from build123d import *

# Parameters (mm, degrees)
F0_W     = 1.25
F0_H     = 45
F1_DEPTH = 10
F0_W_2   = 3.75
F2_DEPTH = 2.5
F3_R     = 2.5
F4_R     = 2.5


with BuildPart() as f1:
    # F0 (on Top) → F1 (new body)
    with BuildSketch(Plane.XY):
        with Locations((-0.625, 45)):
            Rectangle(F0_W, F0_H)
        with Locations((0.625, 45)):
            Rectangle(F0_W, F0_H)
        with Locations((-0.625, 0)):
            Rectangle(F0_W, F0_H)
        with Locations((0.625, 0)):
            Rectangle(F0_W, F0_H)
    extrude(amount=F1_DEPTH)

    # F0 (on Top) → F2 (join)
    with BuildSketch(Plane.XY):
        with Locations((3.125, 0)):
            Rectangle(F0_W_2, F0_H)
        with Locations((-3.125, 0)):
            Rectangle(F0_W_2, F0_H)
        with Locations((0.625, 0)):
            Rectangle(F0_W, F0_H)
        with Locations((-0.625, 0)):
            Rectangle(F0_W, F0_H)
    extrude(amount=F2_DEPTH)

    # F3
    f3_edges = [f1.edges().sort_by_distance(p)[0] for p in [
        (5, 22.5, 1.25),
        (-5, 22.5, 1.25),
        (-5, -22.5, 1.25),
        (5, -22.5, 1.25),
    ]]
    fillet(f3_edges, radius=F3_R)

    # F4
    f4_edges = [f1.edges().sort_by_distance(p)[0] for p in [
        (0, -22.5, 10),
        (0, 67.5, 10),
    ]]
    fillet(f4_edges, radius=F4_R)


solid = f1.part
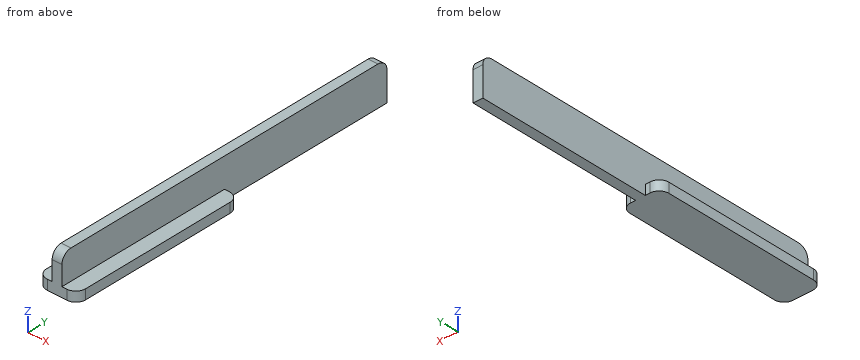
Input: part model. Units: mm. Frame: model coordinates. Round coordinates to 2 decimals unless told otherwise and drop trailing zeros. Loops run counter-clockwise (first coordinate to the right, second up) from the corner with the lowest first, then second, coordinate; pieces in that order, holes last. Notation, with made-up numbers: M 23,-1.75 L 28,-1.75 A30 ccw 28,21.25 Z; hole C 19.25,77.25 d6. An arc over 180 degrees is marked long. Answer as CSV lines item,"result". Start each with the question number.
(1) Section C-C, the plane z = 4.5. Output: boundary loops of the cut face in (x, y).
(2) First-contact query: pin 1 (1.5 mm diameter, centred on y = 48, z = 3.5, fed in from -X); pin 2 (1.1 mm diameter, centred on x = -2, y = 7.5, fed in from +Z); pin 3 (1.4 mm diameter, centred on x = 2, z = 1, fed in from +Y); pin 4 (2 mm diameter, centred on x = 3, y = 56, fed in from -Z). Flat tips, straight axial feed; report the tip coordinate or a pass-through.
(3) Section B-B, the plane x = 3.5. Output: boundary loops of the cut face in (y, z), plus the area to 3 significant figures.
(4) Line query: line 1 (Y direction, x = -2.5, z = 1.25); line 2 (Z direction, x = -1.5, y = 10); line 3 (X direction, y = 38.5, z = 4.75). Output: solid intervals per line, ascending. Write a range as [from, to].
(5) Section A-A, the plane y = 15. Output: boundary loops of the cut face in (x, z).
Values found:
1,outline,"M -1.25,-22.5 L 1.25,-22.5 L 1.25,67.5 L -1.25,67.5 Z"
2,pin 1,"stops at x = -1.25"
2,pin 2,"stops at z = 2.5"
2,pin 3,"stops at y = 22.5"
2,pin 4,"passes through"
3,outline,"M -22.29,0 L 22.29,0 L 22.29,2.5 L -22.29,2.5 Z"
3,area,"111 mm²"
4,line 1,"y = [-22.5, 22.5]"
4,line 2,"z = [0, 2.5]"
4,line 3,"x = [-1.25, 1.25]"
5,outline,"M -5,0 L 5,0 L 5,2.5 L 1.25,2.5 L 1.25,10 L -1.25,10 L -1.25,2.5 L -5,2.5 Z"
